Autodesk Inventor part; units mm, degrees
ref_plane "YZ Plane" through (0, 0, 0) normal (1, 0, 0) x (0, 1, 0)
ref_plane "XZ Plane" through (0, 0, 0) normal (0, 1, 0) x (-1, 0, 0)
ref_plane "XY Plane" through (0, 0, 0) normal (0, 0, 1) x (1, 0, 0)
sketch "Sketch2" plane through (0, 0, 0) normal (0, 1, 0) x (-1, 0, 0)
  line L0 (-22, 25.4) -> (22, 25.4)
  line L1 (22, 25.4) -> (22, -25.4)
  line L2 (22, -25.4) -> (-22, -25.4)
  line L3 (-22, -25.4) -> (-22, 25.4)
  line L4 (-22, 25.4) -> (22, -25.4) construction
  line L5 (22, 25.4) -> (-22, -25.4) construction
  point P0 (0, 0)
  dimension "d0" = 50.8
  dimension "d1" = 44
extrude "Extrusion1" add sketch "Sketch2" along normal blind 25.4
sketch "Sketch3" plane through (-22, 0, 25.4) normal (0, 0, 1) x (1, 0, 0)
  line L0 (0, 25.4) -> (44, 25.4) construction
  line L1 (0, 0) -> (44, 0) construction
  line L2 (44, 0) -> (44, 25.4) construction
  line L3 (44, 25.4) -> (0, 25.4) construction
  line L4 (0, 25.4) -> (0, 0) construction
  line L5 (0, 0) -> (44, 25.4) construction
  line L6 (44, 0) -> (0, 25.4) construction
  line L7 (44, 0) -> (0, 0)
  point P0 (22, 0)
  point P1 (22, 12.7)
hole "Hole1" at (0, 12.7, 25.4) direction (0, 0, -1) diameter 4.134 depth 12.7 tip angle 118
sketch "Sketch4" plane through (0, 25.4, 0) normal (0, 1, 0) x (1, 0, 0)
  line L0 (10, -7.5) -> (10, 7.5) construction
  line L1 (10, 7.5) -> (-10, 7.5) construction
  line L2 (-10, 7.5) -> (-10, -7.5) construction
  line L3 (-10, -7.5) -> (10, -7.5) construction
  line L4 (10, -7.5) -> (-10, 7.5) construction
  line L5 (10, 7.5) -> (-10, -7.5) construction
  circle A0 centre (-10, 7.5) radius 3
  circle A1 centre (10, 7.5) radius 3
  circle A2 centre (10, -7.5) radius 3
  circle A3 centre (-10, -7.5) radius 3
  point P0 (0, 0)
  dimension "d11" = 20
  dimension "d12" = 15
  dimension "d13" = 6
  dimension "d14" = 6
  dimension "d15" = 6
  dimension "d16" = 6
extrude "Extrusion2" cut sketch "Sketch4" against normal blind 5
sketch "Sketch5" plane through (-10, 20.4, 7.5) normal (0, 1, 0) x (1, 0, 0)
  circle A0 centre (0, 15) radius 3
  circle A1 centre (20, 0) radius 3
  circle A2 centre (20, 15) radius 3
  point P0 (10, 7.5)
  point P1 (0, 0)
hole "Hole2" at (-10, 20.4, -7.5) at (-10, 20.4, 7.5) at (10, 20.4, 7.5) at (10, 20.4, -7.5) direction (0, -1, 0) diameter 3.5 end through all
sketch "Sketch8" plane through (-22, 0, -25.4) normal (-1, 0, 0) x (0, 0, 1)
  circle A0 centre (25.4, 19.05) radius 1.75
  line L0 (0, 25.4) -> (50.8, 25.4)
  line L1 (0, 0) -> (0, 25.4)
  circle A1 centre (25.4, 11.1125) radius 1.75
  arc A2 (28.4, 19.05) -> (22.4, 19.05) centre (25.4, 19.05) ccw
  arc A3 (22.4, 11.1125) -> (28.4, 11.1125) centre (25.4, 11.1125) ccw
  line L2 (28.4, 11.1125) -> (28.4, 19.05)
  line L3 (22.4, 19.05) -> (22.4, 11.1125)
  point P0 (25.4, 0)
  dimension "d31" = 3.5
  dimension "d32" = 6.35
  dimension "d33" = 25.4
  dimension "d41" = 3.5
  dimension "d42" = 7.9375
  dimension "d43" = 6
  dimension "d44" = 6
extrude "Extrusion4" cut sketch "Sketch8" against normal blind 22 contours A0 | A1
sketch "Sketch9" plane through (22, 0, -25.4) normal (0, 0, -1) x (-1, 0, 0)
  line L0 (44, 25.4) -> (0, 25.4)
  line L1 (18.698, 25.4) -> (25.302, 25.4)
  line L2 (25.302, 25.4) -> (25.302, 6.35)
  line L3 (25.302, 6.35) -> (18.698, 6.35)
  line L4 (18.698, 6.35) -> (18.698, 25.4)
  line L5 (44, 0) -> (44, 25.4)
  point P0 (22, 0)
  point P1 (22, 6.35)
  dimension "d36" = 6.604
  dimension "d37" = 22
  dimension "d38" = 19.05
extrude "Extrusion5" cut sketch "Sketch9" against normal blind 38.1
extrude "Extrusion6" cut sketch "Sketch8" against normal blind 3
fillet "Fillet1" radius 3.175 2 edges at (3.302, 15.875, 12.7) (-3.302, 15.875, 12.7)
properties part number "Mass 1" material "Steel, Mild"
The listing builds one solid part. Answer for the finished solid, in the listing's coordinates (mm). A direction names the side the tool comes from. Give positions to 0.01 mm unless a question says otherwise; leave off trailing zeros. Order: outer loops, then holes, each group sorted by start corner. A loop starts at its lowest first (then second) coordinate and runs counter-clockwise, first axis right, second up. Notation, with made-up numbers: (55.25, 26.25) - (92.25, 26.25) arc R22 cw to (92.25, 32.25) - close; hole circle Ø10 at (39, 61.25). An arc over 180 degrees is marked (long way). Answer as CSV lines item,"result".
Q1. Determine the mould class of faces 6 (the face through (0, 0, 0)), 7 (the face through (-11.5, 10.1, 8.4)), 8 (the face through (-21, 15, 3)), 9 (the face through (5, 25.4, 0)) for opening direction Y: pulls with the +Y half, pulls with the -Y half, needs draft (parallel to the pull), parting line crosses it, or undercut.
Answer key:
face 6,"pulls with the -Y half"
face 7,"needs draft"
face 8,"undercut"
face 9,"pulls with the +Y half"
Q2. A cutting plane is placed at A-A, the plane x = -10. Determine the outline of the cut face in (y, z), and give its area (3 significant figures).
Answer key:
outline,"(0, -25.4) - (25.4, -25.4) - (25.4, -10.5) - (20.4, -10.5) - (20.4, -9.25) - (0, -9.25) - close; (0, -5.75) - (20.4, -5.75) - (20.4, -4.5) - (25.4, -4.5) - (25.4, 4.5) - (20.4, 4.5) - (20.4, 5.75) - (0, 5.75) - close; (0, 9.25) - (20.4, 9.25) - (20.4, 10.5) - (25.4, 10.5) - (25.4, 25.4) - (0, 25.4) - close; hole circle Ø3.5 at (11.11, 0); hole circle Ø3.5 at (19.05, 0)"
area,"1,070 mm^2"
Q3. A cutting plane is placed at C-C, the plane x = 10. Determine the outline of the cut face in (y, z).
Answer key:
outline,"(0, -25.4) - (25.4, -25.4) - (25.4, -10.5) - (20.4, -10.5) - (20.4, -9.25) - (0, -9.25) - close; (0, -5.75) - (20.4, -5.75) - (20.4, -4.5) - (25.4, -4.5) - (25.4, 4.5) - (20.4, 4.5) - (20.4, 5.75) - (0, 5.75) - close; (0, 9.25) - (20.4, 9.25) - (20.4, 10.5) - (25.4, 10.5) - (25.4, 25.4) - (0, 25.4) - close"
Q4. Which of the six approach directions +Z, -Z, +X, -X, +Y, -Y give full straight-line access (tool end or side, diameter ignored) to faces 1 (the face through (-8, 20.4, -8)), 2 (the face through (8.5, 10.1, 8.4)), 3 (the face through (-3.302, 16, -8)), 4 (the face through (-21, 15, -3)), 5 (the face through (-5, 13, -25.4))?
Answer key:
face 1,"+Y"
face 2,"+Y, -Y"
face 3,"-Z, +Y"
face 4,"-X"
face 5,"-Z, +X, -X, +Y, -Y"
Q5. Each of these flat-tipped pins is pushed along its axis until it touches: pin 1 Ø3 at (x, z) = (-10, -7.5) entering from -Y; pin 2 Ø5.5 at (x, z) = (10, 7.5) entering from +Y; pin 3 Ø3 at (y, z) = (14.5, -1) entering from -X. Where does it stop, or does it pass through?
Answer key:
pin 1,"passes through"
pin 2,"stops at y = 20.4"
pin 3,"stops at x = -19"
Q6. Straight lines are drawn through the part: L1, parallel to Z at x = -10, y = 21.75; L2, parallel to Z at x = 10, y = 6.5; L3, parallel to X at y = 4.25, z = -7.5. For each, find the intervals that lie inside material, in ascending order.
Answer key:
L1,"z = -25.4 to -10.5, -4.5 to 4.5, 10.5 to 25.4"
L2,"z = -25.4 to -9.25, -5.75 to 5.75, 9.25 to 25.4"
L3,"x = -22 to -11.75, -8.25 to 8.25, 11.75 to 22"
Q7. A cutting plane is placed at B-B, the plane z = -7.5. Determine the outline of the cut face in (x, y).
Answer key:
outline,"(-22, 0) - (-11.75, 0) - (-11.75, 20.4) - (-13, 20.4) - (-13, 25.4) - (-22, 25.4) - close; (-8.25, 0) - (8.25, 0) - (8.25, 20.4) - (7, 20.4) - (7, 25.4) - (3.3, 25.4) - (3.3, 6.35) - (-3.3, 6.35) - (-3.3, 25.4) - (-7, 25.4) - (-7, 20.4) - (-8.25, 20.4) - close; (11.75, 0) - (22, 0) - (22, 25.4) - (13, 25.4) - (13, 20.4) - (11.75, 20.4) - close"
Q8. A cutting plane is placed at D-D, the plane y = 11.75. Determine the outline of the cut face in (x, z) (3 decimals).
Answer key:
outline,"(-22, -25.4) - (-3.302, -25.4) - (-3.302, -1.63) - (-19, -1.63) - (-19, -3) - (-22, -3) - close; (-22, 3) - (-19, 3) - (-19, 1.63) - (-3.302, 1.63) - (-3.302, 9.525) arc R3.175 cw to (-1.836, 12.201) - (-1.836, 25.4) - (-22, 25.4) - close; (1.836, 12.201) arc R3.175 cw to (3.302, 9.525) - (3.302, -25.4) - (22, -25.4) - (22, 25.4) - (1.836, 25.4) - close; hole circle Ø3.5 at (-10, -7.5); hole circle Ø3.5 at (-10, 7.5); hole circle Ø3.5 at (10, -7.5); hole circle Ø3.5 at (10, 7.5)"
